Read the model definition and answer for the solid it produces. Units are mm, in the model's axes. A direction names the side the tool comes from. Coordinates: 2 decimals unless noted, no trailing zeros. Order: outer loops, then holes, each group sorted by start corner. A loop starts at its lowest first (then second) coordinate and runs counter-clockwise, first axis right, second up. Notation, with made-up numbers: M 29,-37 L 75,-37 A31 ccw 75,-8 Z; hole C 9.25,22 d7. An arc over 180 degrees is marked long. Put each result on its own line as item: value.
from build123d import *

# Parameters (mm, degrees)
F1_DEPTH  = 7.5
F2_W      = 2.6
F2_H      = 4.75
F0_R      = 18.75
F4_DEPTH  = 2.375
F8_R      = 4
F9_W      = 29.1621480137
F9_H      = 87.7830125391
F9_W_2    = 6.8209778983
F10_DEPTH = 60.1


# Not quite as in the source:
# - a feature names something its author has since deleted; it is built from what else it names


with BuildPart() as f1:
    # F0 (on Right) → F1 (new body)
    with BuildSketch(Plane.YZ):
        with BuildLine():
            Line((-27.5, -30.8578620553), (-27.5, 35))
            Line((-27.5, 35), (-35, 35))
            Line((-35, 35), (-35, -33.3578620553))
            ThreePointArc((-35, -33.3578620553), (-32.0710678119, -40.4289298672), (-25, -43.3578620553))
            Line((-25, -43.3578620553), (25, -43.3578620553))
            ThreePointArc((25, -43.3578620553), (32.0710678119, -40.4289298672), (35, -33.3578620553))
            Line((35, -33.3578620553), (35, 35))
            Line((35, 35), (27.5, 35))
            Line((27.5, 35), (27.5, -30.8578620553))
            ThreePointArc((27.5, -30.8578620553), (26.0355339059, -34.3933959612), (22.5, -35.8578620553))
            Line((22.5, -35.8578620553), (-22.5, -35.8578620553))
            ThreePointArc((-22.5, -35.8578620553), (-26.0355339059, -34.3933959612), (-27.5, -30.8578620553))
        make_face()
    extrude(amount=F1_DEPTH)

    # F3: sweep along a path in F0
    with BuildLine(Plane.YZ) as f3_path:
        Line((27.5, 35), (27.5, -30.8578620553))
        ThreePointArc((27.5, -30.8578620553), (26.0355339059, -34.3933959612), (22.5, -35.8578620553))
        Line((22.5, -35.8578620553), (-22.5, -35.8578620553))
        ThreePointArc((-22.5, -35.8578620553), (-26.0355339059, -34.3933959612), (-27.5, -30.8578620553))
        Line((-27.5, -30.8578620553), (-27.5, 35))
    # F2 (on face) → F3 (sweep, cut)
    with BuildSketch(Plane.XY.offset(35)):
        with Locations((3.675, 29.875)):
            Rectangle(F2_W, F2_H)
    sweep(path=f3_path.line, mode=Mode.SUBTRACT)

    # F0 (on Right) → F4 (join)
    with BuildSketch(Plane.YZ):
        with BuildLine():
            Line((27.5, 35), (-27.5, 35))
            Line((-27.5, 35), (-27.5, -30.8578620553))
            ThreePointArc((-27.5, -30.8578620553), (-26.0355339059, -34.3933959612), (-22.5, -35.8578620553))
            Line((-22.5, -35.8578620553), (22.5, -35.8578620553))
            ThreePointArc((22.5, -35.8578620553), (26.0355339059, -34.3933959612), (27.5, -30.8578620553))
            Line((27.5, -30.8578620553), (27.5, 35))
        make_face()
        with Locations((2, 3)):
            Circle(F0_R, mode=Mode.SUBTRACT)
    extrude(amount=F4_DEPTH)

    # F6 (on offset) → F7 (revolve)
    with BuildSketch(Plane.XY.offset(1)):
        Polygon((0, 22), (0, 25), (-22.6, 35), (-22.6, 32), align=None)
    revolve(axis=Axis((0, 2, 3), (1, 0, 0)))

    # F8
    f8_edges = [f1.edges().sort_by_distance(p)[0] for p in [
        (6.2375, -27.5, 35),
        (6.2375, 27.5, 35),
    ]]
    fillet(f8_edges, radius=F8_R)

    # F9 (on offset) → F10 (cut, symmetric)
    with BuildSketch(Plane.XY.offset(1)):
        with Locations((-14.5810740069, 1.1862572283)):
            Rectangle(F9_W, F9_H)
        with Locations((7.2658261051, 1.1862572283)):
            Rectangle(F9_W_2, F9_H)
    extrude(amount=F10_DEPTH, both=True, mode=Mode.SUBTRACT)


solid = f1.part
Q1. For a pull along Y with two mould halves and no side action, classify faces 1 (the face through (1.9, -32.1, -40.4)), 2 (the face through (3.105, -29.318, -37.828)), 3 (the face through (2, 35, 0)) as +Y half, -Y half, draft (parallel to the pull), parting line (faces both ways), or undercut.
Answers below:
face 1: -Y half
face 2: undercut
face 3: +Y half
Q2. A tool of negligible diameter and unlimited length cuts with its end or side. For faces 4 (the face through (0, -16, -4)), 5 (the face through (3.105, 29.47, -37.676)), from which of +Z, -Z, +X, -X, +Y, -Y can it reach the whole face along a straight path? Write none if from no direction.
Answers below:
face 4: +Z, -Z, -X, +Y, -Y
face 5: +Z, +X
Q3. Consider line 1 along Y through (x, z) = (0.7, 3.5); line 2 along Y through (x, z) = (3.45, -24); line 3 along Z through (x, y) = (1.8, 2). Determine where each line is inside the solid, lowest interval first.
Answers below:
line 1: y = -35 to -16.74, 20.74 to 35
line 2: y = -35 to -32.25, 32.25 to 35
line 3: z = -43.36 to -15.75, 21.75 to 35
Q4. Find section D-D on z = -27. Write down the section's boundary in (x, y) (3 decimals).
Answers below:
outline: M 0,-35 L 3.855,-35 L 3.855,-32.25 L 2.375,-32.25 L 2.375,32.25 L 3.855,32.25 L 3.855,35 L 0,35 Z
Q5. Find section A-A on y = 2. Write down the section's boundary in (x, z) (3 decimals).
Answers below:
outline: M 0,-43.358 L 3.855,-43.358 L 3.855,-40.608 L 2.375,-40.608 L 2.375,-15.75 L 0,-15.75 Z; M 0,21.75 L 2.375,21.75 L 2.375,35 L 0,35 Z
Q6. Find section B-B on x = 1.1. Write down the section's boundary in (y, z).
Answers below:
outline: M -35,-33.36 A10 ccw -25,-43.36 L 25,-43.36 A10 ccw 35,-33.36 L 35,35 L -35,35 Z; hole C 2,3 d37.5
Q7. Find section C-C on z = 3. Write down the section's boundary in (x, y) (3 decimals), plus the area to 3 significant figures.
Answers below:
outline: M 0,-35 L 3.855,-35 L 3.855,-32.25 L 2.375,-32.25 L 2.375,-16.75 L 0,-16.75 Z; M 0,20.75 L 2.375,20.75 L 2.375,32.25 L 3.855,32.25 L 3.855,35 L 0,35 Z
area: 85.3 mm^2
Q8. Given pin 1 (0.7 mm diameter, centred on x = 3, y = -5, fed in from +Z); pin 2 (4 mm diameter, centred on y = 10.5, z = 27, fed in from +X) (3 decimals), each flat-ended and moving along its own axis, determine where each tip first touches the part or whether it passes through.
Answers below:
pin 1: stops at z = -40.61
pin 2: stops at x = 2.375
